from build123d import *

# Parameters (mm, degrees)
F3_DEPTH = 12.7


with BuildPart() as f2:
    # F2: sweep along a path in F0
    with BuildLine(Plane.XZ) as f2_path:
        ThreePointArc((0, 76.2), (53.881537, 53.881537), (76.2, 0))
    # F1 (on Top) → F2 (sweep)
    with BuildSketch(Plane.XY):
        with BuildLine():
            Line((52.193511, 0), (75.958066, 0))
            ThreePointArc((75.958066, 0), (64.075788, 8.704073), (52.193511, 0))
        make_face()
    sweep(path=f2_path.line)

    # F0 (on Front) → F3 (join)
    with BuildSketch(Plane.XZ):
        with BuildLine():
            Line((0, 76.2), (0, 0))
            Line((0, 0), (76.2, 0))
            ThreePointArc((76.2, 0), (53.881537, 53.881537), (0, 76.2))
        make_face()
        with BuildLine():
            ThreePointArc((0, 76.2), (53.881537, 53.881537), (76.2, 0))
            Line((76.2, 0), (101.6, 0))
            Line((101.6, 0), (101.6, 76.2))
            Line((101.6, 76.2), (0, 76.2))
        make_face()
    extrude(amount=F3_DEPTH)


solid = f2.part
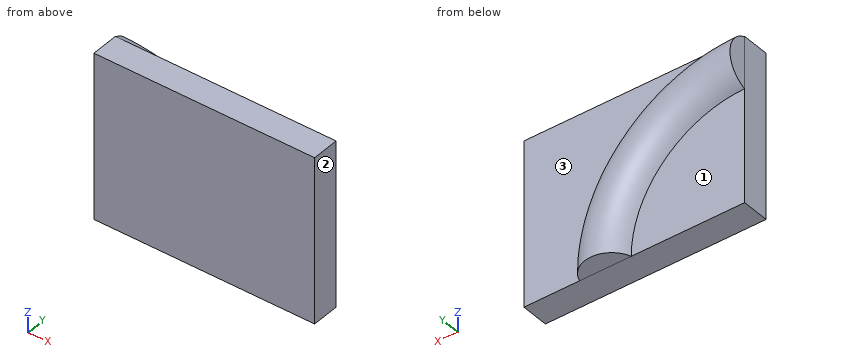
Geometry: final body of the model. Coordinates: model frame, mm. Face numbers are marked on the shaded views. A direction names the side the tool comes from. Round coordinates to 2 decimals unless told otherwise and drop trailing zeros. Loops run counter-clockwise (first coordinate to the right, second up) from the corner with the lowest first, then second, coordinate; pieces in that order, holes last.
Q1. Material intervals for L1, parallel to Y at x = 17, z = 49; L2, parallel to Y at x = 52.5, z = 34.5; L3, parallel to X at y = 1.5, z = 27, sorted ascending.
Q2. Section B-B on y = 4.75. Return loops of the section in (x, z).
Q3. Section A-A on x = 81. Return loops of the section in (y, z), plus the area to 3 significant figures.
Q4. Access query for the marked faces 1, 2 and 3. Directions: +Z, -Z, +X, -X, +Y, -Y. A direction counts if a zero-diameter tool reaches every point of the face in a straight line with its end or side. Return the directions, or none.
Q5. Pin query (flat end, axial travel): P1, Ø2, axis at y = 4, z = 17, coming from the +X side; P2, Ø6, axis at x = 74.5, z = 59, coming from the +Y side; P3, Ø2, axis at x = 49, z = 43.5, coming from the +Y side. Return the tip coordinate at first contact, or that it passes through.
Evaluation:
1. L1: y = -12.7 to 0
1. L2: y = -12.7 to 8.64
1. L3: x = 45.35 to 70.37
2. outline: (0, 54.97) arc R54.97 cw to (54.97, 0) - (73.18, 0) arc R73.18 ccw to (0, 73.18) - close
3. outline: (-12.7, 0) - (0, 0) - (0, 76.2) - (-12.7, 76.2) - close
3. area: 968 mm2
4. face 1: -Z, -X, +Y
4. face 2: +Z, -Z, +X, +Y, -Y
4. face 3: +Z, +X, +Y
5. P1: stops at x = 72.62
5. P2: stops at y = 0
5. P3: stops at y = 8.7
